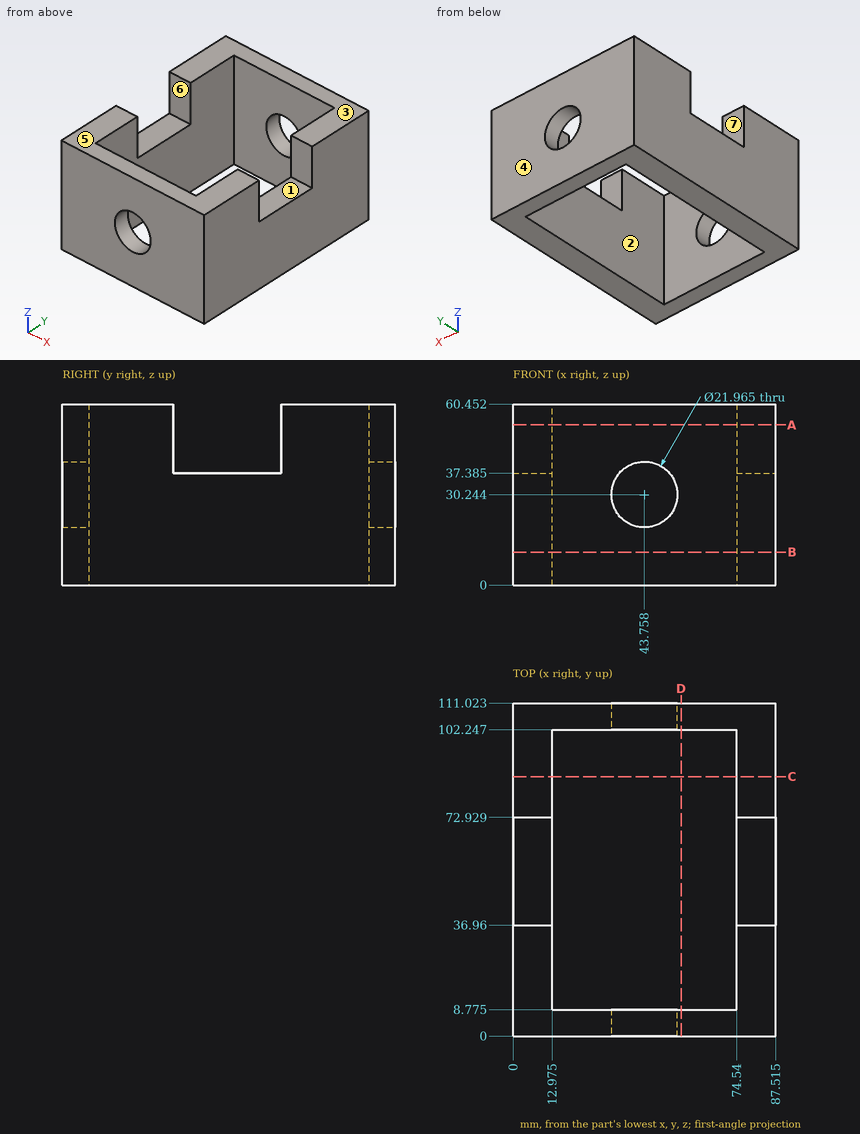
The figure shows three views and two pictorial views of one solid part (mm, origin at its lowest corner). Answer the questions. A direction names the side the tool comes from. Round coordinates to 2 decimals unless told otherwise and drop trailing zeros. Write each loop counter-clockwise with the first axis right and the second up, starting at its lowest first coordinate (ties: lowest second). Pieces come first, ordered by that corner, then holes. Notation, with made-up numbers: (0.25, -35) -> (18.25, -35) arc R8 cw to (18.25, -28) -> close; hole circle Ø7 at (34.5, -30.5). An arc over 180 degrees is marked (long way). Write each question's results on one line, items separated by ' | '.
Q1. Section A-A, the plane z = 53.5 is taken. Write down the section's boundary in (x, y) (1 decimal), then the cut area to 3 significant figures.
Data:
outline: (0, 0) -> (87.5, 0) -> (87.5, 37) -> (74.5, 37) -> (74.5, 8.8) -> (13, 8.8) -> (13, 37) -> (0, 37) -> close; (0, 72.9) -> (13, 72.9) -> (13, 102.2) -> (74.5, 102.2) -> (74.5, 72.9) -> (87.5, 72.9) -> (87.5, 111) -> (0, 111) -> close | area: 3,030 mm^2
Q2. Section B-B, the plane z = 11 is taken. Write down the section's boundary in (x, y) (1 decimal), then the cut area to 3 significant figures.
Data:
outline: (0, 0) -> (87.5, 0) -> (87.5, 111) -> (0, 111) -> close; hole (13, 8.8) -> (74.5, 8.8) -> (74.5, 102.2) -> (13, 102.2) -> close | area: 3,960 mm^2
Q3. Which of the six approach directions +Z, -Z, +X, -X, +Y, -Y give full straight-line access (tool end or side, diameter ignored) to the marked faces 1, 2 and 3?
Data:
face 1: +Z, +X, -X | face 2: +Z, -Z | face 3: +Z, +X, -X, +Y, -Y
Q4. Section C-C, the plane y = 86.5 is taken. Write down the section's boundary in (x, z) (1 decimal).
Data:
outline: (0, 0) -> (13, 0) -> (13, 60.5) -> (0, 60.5) -> close; (74.5, 0) -> (87.5, 0) -> (87.5, 60.5) -> (74.5, 60.5) -> close
Q5. Section D-D, the plane x = 56 is taken. Write down the section's boundary in (y, z) (1 decimal), then the cut area to 3 significant figures.
Data:
outline: (0, 0) -> (8.8, 0) -> (8.8, 60.5) -> (0, 60.5) -> close; (102.2, 0) -> (111, 0) -> (111, 60.5) -> (102.2, 60.5) -> close | area: 1,060 mm^2
Q6. Straight lines are drawn through the part: line 1 along Y through (x, z) = (21, 32) (1 decimal); line 2 along X through (y, z) = (100.5, 22) (1 decimal); line 3 along Y through (x, z) = (6, 52). For each, find the intervals that lie inside material, in ascending order. Write a range as [from, to].
Data:
line 1: [0, 8.8], [102.2, 111] | line 2: [0, 13], [74.5, 87.5] | line 3: [0, 36.96], [72.93, 111.02]
Q7. Determine the mould class of the marked faces 4, 5, 6 and 7 for opening direction Y: released by +Y, released by -Y, zero draft, split by the parting line, or undercut.
Data:
face 4: released by +Y | face 5: zero draft | face 6: undercut | face 7: undercut
Q8. Flat-ended cylindrical pins translate along their axes: P1, Ø6.5, axis at x = 81.5, y = 61, coming from the +Z side (1 decimal); P2, Ø10, axis at x = 66.5, y = 62, coming from the +Z side. Find the tip coordinate at first contact, or state that the pin passes through.
Data:
P1: z = 37.4 | P2: through
